from build123d import *

# Parameters (mm, degrees)
BOSS_EXTRUDE1_DEPTH = 0.254
SKETCH2_R           = 4.699
CUT_EXTRUDE1_DEPTH  = 1.254
SKETCH3_W           = 2.54
SKETCH3_H           = 0.635
CUT_EXTRUDE2_DEPTH  = 1.254
CUT_EXTRUDE4_DEPTH  = 1.254
CUT_EXTRUDE5_DEPTH  = 1.254


with BuildPart() as part:
    # Sketch1 → Boss-Extrude1 (new body)
    with BuildSketch(Plane.XY):
        with BuildLine():
            Line((67.21146711, 76.191723231), (8.696654013, 17.676910134))
            Line((8.696654013, 17.676910134), (7.228954972, 14.133571205))
            ThreePointArc((7.228954972, 14.133571205), (14.666587579, 6.075099489), (15.105587123, -4.88230096))
            Line((15.105587123, -4.88230096), (18.648926052, -6.35))
            Line((18.648926052, -6.35), (101.401368334, -6.35))
            ThreePointArc((101.401368334, -6.35), (93.866160503, 38.880636728), (67.21146711, 76.191723231))
        make_face()
        with BuildLine():
            Line((88.672924278, 6.35), (27.86051193, 6.35))
            ThreePointArc((27.86051193, 6.35), (26.399857642, 10.93517908), (24.190484974, 15.210228852))
            Line((24.190484974, 15.210228852), (67.191354125, 58.211098004))
            ThreePointArc((67.191354125, 58.211098004), (82.13289044, 34.020557137), (88.672924278, 6.35))
        make_face(mode=Mode.SUBTRACT)
    extrude(amount=BOSS_EXTRUDE1_DEPTH)

    # Sketch2 → Cut-Extrude1 (cut, through all)
    with BuildSketch(Plane.XY.offset(0.254)):
        with Locations((22.225, 0)):
            Circle(SKETCH2_R)
        with Locations((36.195, 0)):
            Circle(SKETCH2_R)
        with Locations((61.722, 0)):
            Circle(SKETCH2_R)
        with Locations((75.692, 0)):
            Circle(SKETCH2_R)
        with Locations((95.25, 0)):
            Circle(SKETCH2_R)
        with Locations((15.715448212, 15.715448212)):
            Circle(SKETCH2_R)
        with Locations((25.593729945, 25.593729945)):
            Circle(SKETCH2_R)
        with Locations((43.644044748, 43.644044748)):
            Circle(SKETCH2_R)
        with Locations((53.522326482, 53.522326482)):
            Circle(SKETCH2_R)
        with Locations((92.004434954, 24.652514046)):
            Circle(SKETCH2_R)
        with Locations((82.48891971, 47.625)):
            Circle(SKETCH2_R)
        with Locations((67.351920908, 67.351920908)):
            Circle(SKETCH2_R)
    extrude(amount=-CUT_EXTRUDE1_DEPTH, mode=Mode.SUBTRACT)

    # Sketch3 → Cut-Extrude2 (cut, through all)
    with BuildSketch(Plane.XY.offset(0.254)):
        Polygon((15.266435406, 24.246691527), (17.06248663, 26.042742751), (17.511499436, 25.593729945), (15.715448212, 23.797678721), align=None)
        Polygon((44.991083167, 53.971339288), (43.195031942, 52.175288063), (43.644044748, 51.726275257), (45.440095973, 53.522326482), align=None)
        with Locations((29.21, -6.0325)):
            Rectangle(SKETCH3_W, SKETCH3_H)
        with Locations((68.707, -6.0325)):
            Rectangle(SKETCH3_W, SKETCH3_H)
        Polygon((29.230733674, 38.210989795), (31.026784898, 40.007041019), (31.475797704, 39.558028213), (29.67974648, 37.761976989), align=None)
        Polygon((56.845021246, 65.825277367), (55.048970022, 64.029226143), (55.497982828, 63.580213337), (57.294034052, 65.376264561), align=None)
        with Locations((48.9585, -6.0325)):
            Rectangle(SKETCH3_W, SKETCH3_H)
        with Locations((85.471, -6.0325)):
            Rectangle(SKETCH3_W, SKETCH3_H)
        Polygon((99.935462164, 14.437711971), (100.266998693, 11.919442024), (101.526133667, 12.085210288), (101.194597138, 14.603480236), align=None)
        Polygon((93.765504959, 37.464305742), (94.938831965, 37.950313702), (93.966816047, 40.296967714), (92.793489041, 39.810959755), align=None)
        Polygon((79.327792988, 62.471156422), (80.874047017, 60.456038938), (81.88160576, 61.229165953), (80.33535173, 63.244283437), align=None)
        Polygon((13.593916116, 7.005422516), (14.565932035, 4.658768503), (15.739259041, 5.144776462), (14.767243123, 7.491430475), align=None)
    extrude(amount=-CUT_EXTRUDE2_DEPTH, mode=Mode.SUBTRACT)

    # Sketch6 → Cut-Extrude4 (cut, through all)
    with BuildSketch(Plane.XY.offset(0.254)):
        with BuildLine():
            Line((12.392753447, 19.038142977), (22.27103518, 28.91642471))
            ThreePointArc((22.27103518, 28.91642471), (28.91642471, 28.91642471), (28.91642471, 22.27103518))
            Line((28.91642471, 22.27103518), (19.038142977, 12.392753447))
            ThreePointArc((19.038142977, 12.392753447), (12.392753447, 12.392753447), (12.392753447, 19.038142977))
        make_face()
        with BuildLine():
            Line((22.225, 4.699), (36.195, 4.699))
            ThreePointArc((36.195, 4.699), (40.894, 0), (36.195, -4.699))
            Line((36.195, -4.699), (22.225, -4.699))
            ThreePointArc((22.225, -4.699), (17.526, 0), (22.225, 4.699))
        make_face()
        with BuildLine():
            Line((61.722, 4.699), (75.692, 4.699))
            ThreePointArc((75.692, 4.699), (80.391, 0), (75.692, -4.699))
            Line((75.692, -4.699), (61.722, -4.699))
            ThreePointArc((61.722, -4.699), (57.023, 0), (61.722, 4.699))
        make_face()
        with BuildLine():
            ThreePointArc((99.949, 0), (99.093922449, 13.045962386), (96.543320412, 25.868704739))
            ThreePointArc((96.543320412, 25.868704739), (90.788244261, 29.191399504), (87.465549496, 23.436323353))
            ThreePointArc((87.465549496, 23.436323353), (89.776323642, 11.819277232), (90.551, 0))
            ThreePointArc((90.551, 0), (95.25, -4.699), (99.949, 0))
        make_face()
        with BuildLine():
            ThreePointArc((86.558373083, 49.9745), (79.294873009, 60.845096068), (70.674615673, 70.674615673))
            ThreePointArc((70.674615673, 70.674615673), (64.029226143, 70.674615673), (64.029226143, 64.029226143))
            ThreePointArc((64.029226143, 64.029226143), (71.838938317, 55.123956158), (78.419466338, 45.2755))
            ThreePointArc((78.419466338, 45.2755), (84.83841971, 43.555546628), (86.558373083, 49.9745))
        make_face()
    extrude(amount=-CUT_EXTRUDE4_DEPTH, mode=Mode.SUBTRACT)

    # Sketch5 → Cut-Extrude5 (cut, through all)
    with BuildSketch(Plane.XY.offset(0.254)):
        Polygon((53.881536726, 44.901280605), (64.119028704, 55.138772583), (55.138772583, 64.119028704), (44.901280605, 53.881536726), align=None)
    extrude(amount=-CUT_EXTRUDE5_DEPTH, mode=Mode.SUBTRACT)


solid = part.part
Geometry check sheet. Reference: the model listing, model coordinates, mm. Coordinates: 2 decimals unless noted, no trailing zeros. Order: outer loops, then holes, each group sorted by start corner. A loop starts at its lowest first (then second) coordinate and runs counter-clockwise, first axis right, second up. Notation, with made-up numbers: (21, -2.5) - (53, -2.5) arc R19 ccw to (53, 17.5) - close; hole circle Ø2 at (31.25, 43.5). An arc over 180 degrees is marked (long way). One line per item, written item: value.
(1) Sectioned sample at B-B (x = 72). Enter the section's corners in (y, z), and give its area (3 significant figures).
Data:
outline: (-6.35, 0) - (-4.7, 0) - (-4.7, 0.25) - (-6.35, 0.25) - close; (4.7, 0) - (6.35, 0) - (6.35, 0.25) - (4.7, 0.25) - close; (52.15, 0) - (54.91, 0) - (54.91, 0.25) - (52.15, 0.25) - close; (69.32, 0) - (71.68, 0) - (71.68, 0.25) - (69.32, 0.25) - close
area: 2.14 mm^2
(2) Sectioned sample at C-C (x = 52.5). Enter the section's corners in (y, z), and give its area (3 significant figures).
Data:
outline: (-6.35, 0) - (6.35, 0) - (6.35, 0.25) - (-6.35, 0.25) - close; (43.52, 0) - (46.28, 0) - (46.28, 0.25) - (43.52, 0.25) - close
area: 3.93 mm^2
(3) Sectioned sample at D-D (z = 0.15). Count the separate pieces of the cut face and the enclosed holes in it, and give its area (3 significant figures).
Data:
separate pieces: 1
enclosed holes: 6
area: 1,550 mm^2
(4) Depth check by flat-ended pin: pin 1 Ø5.5 at (x, y) = (43.64, 43.64) entering from +Z. Enter the tip coordinate at first touch or a pass-through.
Data:
pin 1: passes through
(5) Thickness scan on probe 1 along X at (y, z) = (15, 0.05); probe 2 along X at (y, z) = (45.5, 0.15); probe 3 along Y at (x, z) = (42, 0.1). Record the ranges inside material, lowest first. Write a range as from..to.
Data:
probe 1: x = 7.59..11.07, 21.65..24.32, 87.63..89.3, 98.82..100.49
probe 2: x = 36.52..39.33, 47.96..53.28, 76.37..78.29, 86.68..90.84
probe 3: y = -6.35..6.35, 33.02..39.24, 48.05..50.98
(6) Sectioned sample at A-A (y = 10). Enter the section's corners in (x, z), and give its area (3 significant figures).
Data:
outline: (12.33, 0) - (26.77, 0) - (26.77, 0.25) - (12.33, 0.25) - close; (88.34, 0) - (90, 0) - (90, 0.25) - (88.34, 0.25) - close; (99.45, 0) - (101.11, 0) - (101.11, 0.25) - (99.45, 0.25) - close
area: 4.51 mm^2
